```python
from build123d import *

# Parameters (mm, degrees)
BOSS_EXTRUDE33_DEPTH = 5
BOSS_EXTRUDE34_START = 5
BOSS_EXTRUDE34_DEPTH = 1
BOSS_EXTRUDE35_START = -4
BOSS_EXTRUDE35_DEPTH = 4
CUT_EXTRUDE2_DEPTH   = 35.891044696
CUT_EXTRUDE3_DEPTH   = 30.173146899
SKETCH22_W           = 13.5
SKETCH22_H           = 2
BOSS_EXTRUDE37_DEPTH = 1.75
SKETCH23_W           = 3
SKETCH23_H           = 3
BOSS_EXTRUDE38_DEPTH = 1.75
CUT_EXTRUDE4_DEPTH   = 3
CUT_EXTRUDE5_DEPTH   = 17.5


with BuildPart() as part:
    # lid → Boss-Extrude33 (new body)
    with BuildSketch(Plane(origin=(0, 0, 0), x_dir=(1, 0, 0), z_dir=(0, 1, 0))):
        with BuildLine():
            Line((-10.25, 23.85), (12.5, 23.85))
            ThreePointArc((12.5, 23.85), (13.207106781, 23.557106781), (13.5, 22.85))
            Line((13.5, 22.85), (13.5, -7.9))
            ThreePointArc((13.5, -7.9), (13.207106781, -8.607106781), (12.5, -8.9))
            Line((12.5, -8.9), (-10.25, -8.9))
            ThreePointArc((-10.25, -8.9), (-10.957106781, -8.607106781), (-11.25, -7.9))
            Line((-11.25, -7.9), (-11.25, 22.85))
            ThreePointArc((-11.25, 22.85), (-10.957106781, 23.557106781), (-10.25, 23.85))
        make_face()
        with BuildLine():
            Line((-10.5, 22.6), (-10.5, -7.65))
            ThreePointArc((-10.5, -7.65), (-10.353553391, -8.003553391), (-10, -8.15))
            Line((-10, -8.15), (12.25, -8.15))
            ThreePointArc((12.25, -8.15), (12.603553391, -8.003553391), (12.75, -7.65))
            Line((12.75, -7.65), (12.75, 22.6))
            ThreePointArc((12.75, 22.6), (12.603553391, 22.953553391), (12.25, 23.1))
            Line((12.25, 23.1), (-10, 23.1))
            ThreePointArc((-10, 23.1), (-10.353553391, 22.953553391), (-10.5, 22.6))
        make_face(mode=Mode.SUBTRACT)
    extrude(amount=BOSS_EXTRUDE33_DEPTH)

    # lid_5 → Boss-Extrude34 (add)
    with BuildSketch(Plane(origin=(0, 0, 0), x_dir=(1, 0, 0), z_dir=(0, 1, 0)).offset(BOSS_EXTRUDE34_START)):
        with BuildLine():
            Line((12.5, 23.85), (-10.25, 23.85))
            ThreePointArc((-10.25, 23.85), (-10.957106781, 23.557106781), (-11.25, 22.85))
            Line((-11.25, 22.85), (-11.25, -7.9))
            ThreePointArc((-11.25, -7.9), (-10.957106781, -8.607106781), (-10.25, -8.9))
            Line((-10.25, -8.9), (12.5, -8.9))
            ThreePointArc((12.5, -8.9), (13.207106781, -8.607106781), (13.5, -7.9))
            Line((13.5, -7.9), (13.5, 22.85))
            ThreePointArc((13.5, 22.85), (13.207106781, 23.557106781), (12.5, 23.85))
        make_face()
    extrude(amount=BOSS_EXTRUDE34_DEPTH)

    # lid_7 → Boss-Extrude35 (add)
    with BuildSketch(Plane(origin=(0, 0, 0), x_dir=(1, 0, 0), z_dir=(0, 1, 0)).offset(BOSS_EXTRUDE35_START)):
        with BuildLine():
            Line((-10.25, 23.85), (12.5, 23.85))
            ThreePointArc((12.5, 23.85), (13.207106781, 23.557106781), (13.5, 22.85))
            Line((13.5, 22.85), (13.5, -7.9))
            ThreePointArc((13.5, -7.9), (13.207106781, -8.607106781), (12.5, -8.9))
            Line((12.5, -8.9), (-10.25, -8.9))
            ThreePointArc((-10.25, -8.9), (-10.957106781, -8.607106781), (-11.25, -7.9))
            Line((-11.25, -7.9), (-11.25, 22.85))
            ThreePointArc((-11.25, 22.85), (-10.957106781, 23.557106781), (-10.25, 23.85))
        make_face()
        with BuildLine():
            Line((-10.5, 22.6), (-10.5, -7.65))
            ThreePointArc((-10.5, -7.65), (-10.353553391, -8.003553391), (-10, -8.15))
            Line((-10, -8.15), (12.25, -8.15))
            ThreePointArc((12.25, -8.15), (12.603553391, -8.003553391), (12.75, -7.65))
            Line((12.75, -7.65), (12.75, 22.6))
            ThreePointArc((12.75, 22.6), (12.603553391, 22.953553391), (12.25, 23.1))
            Line((12.25, 23.1), (-10, 23.1))
            ThreePointArc((-10, 23.1), (-10.353553391, 22.953553391), (-10.5, 22.6))
        make_face(mode=Mode.SUBTRACT)
    extrude(amount=BOSS_EXTRUDE35_DEPTH)

    # Sketch21 → Cut-Extrude2 (cut, through all)
    with BuildSketch(Plane(origin=(13.5, 0, 0), x_dir=(0, 0, -1), z_dir=(1, 0, 0))):
        with BuildLine():
            Line((4.05, 0), (4.05, -4))
            Line((4.05, -4), (10.05, -4))
            Line((10.05, -4), (10.05, 0))
            ThreePointArc((10.05, 0), (7.05, 3), (4.05, 0))
        make_face()
    extrude(amount=-CUT_EXTRUDE2_DEPTH, mode=Mode.SUBTRACT)

    # Sketch20 → Cut-Extrude3 (cut, through all)
    with BuildSketch(Plane(origin=(0, 6, 0), x_dir=(1, 0, 0), z_dir=(0, 1, 0))):
        with BuildLine():
            Line((-6.5, -3), (8.5, -3))
            ThreePointArc((8.5, -3), (10, -4.5), (8.5, -6))
            Line((8.5, -6), (-6.5, -6))
            ThreePointArc((-6.5, -6), (-8, -4.5), (-6.5, -3))
        make_face()
    extrude(amount=-CUT_EXTRUDE3_DEPTH, mode=Mode.SUBTRACT)

    # Sketch22 → Boss-Extrude37 (add)
    with BuildSketch(Plane(origin=(0, 0, 8.15), x_dir=(-1, 0, 0), z_dir=(0, 0, -1))):
        with Locations((-0.75, -3)):
            Rectangle(SKETCH22_W, SKETCH22_H)
    extrude(amount=BOSS_EXTRUDE37_DEPTH)

    # Sketch23 → Boss-Extrude38 (add)
    with BuildSketch(Plane.XY.offset(-23.1)):
        with Locations((-7.5, -2.5)):
            Rectangle(SKETCH23_W, SKETCH23_H)
        with Locations((9.75, -2.5)):
            Rectangle(SKETCH23_W, SKETCH23_H)
    extrude(amount=BOSS_EXTRUDE38_DEPTH)

    # Sketch24 → Cut-Extrude4 (cut)
    with BuildSketch(Plane.ZY.offset(-8.25)):
        Polygon((-23.1, -4), (-21.35, -1), (-21.35, -4), align=None)
    extrude(amount=-CUT_EXTRUDE4_DEPTH, mode=Mode.SUBTRACT)

    # Sketch24_2 → Cut-Extrude5 (cut)
    with BuildSketch(Plane.ZY.offset(-8.25)):
        Polygon((-23.1, -4), (-21.35, -1), (-21.35, -4), align=None)
    extrude(amount=CUT_EXTRUDE5_DEPTH, mode=Mode.SUBTRACT)


solid = part.part
```
Model file for the job. Use its own axes, mm. A direction names the side the tool comes from. Coordinates: 2 decimals unless noted, no trailing zeros. Write each loop counter-clockwise with the first axis right and the second up, starting at its lowest first coordinate (ties: lowest second). Pieces come first, ordered by that corner, then holes. Notation, with made-up numbers: (3.5, 9.25) - (18.5, 9.25) arc R16 ccw to (18.5, 24.25) - close; hole circle Ø7 at (34, 75). An arc over 180 degrees is marked (long way). One line per item, written item: value. Start each with the question number.
1. Slice it at D-D (z = -7.05). Write the cut outline in (x, y), plus the area to 4 significant figures.
2. Mould opens along Z. For faces 1 (the cylindrical face through (-10.965, 0.93, -23.549)), 2 (the cylindrical face through (-10.949, 0.93, 8.615)), 3 (the flat face through (-9, -1.9, -22.6)), 4 (the flat face through (13.5, 3.2, -7.7)) say: released by +Z, released by -Z, zero draft, split by the parting line, or undercut.
3. Probe line 1 (X direction, y = 3.25, z = -8); line 2 (Z direction, x = 2, y = -1.5); line 3 (Z direction, x = 4.75, y = -2.75). List the from-to ranges inside material, lowest first. Write a range as from..to.
4. Slice it at C-C (z = 4.5). Write the cut outline in (x, y), plus the area to 4 significant figures.
5. Tool access for faces 5 (the flat face through (1, 1, -23.1)), 6 (the flat face through (1, 1, -23.85)), 7 (the flat face through (1.2, -4, -23.6)), 8 (the flat face through (0.9, 5.5, 3)), 9 (the flat face through (-10.5, 3.4, -7.7)): list every direction of +Z, -Z, +X, -X, +Y, -Y with a clear straight run to the whole face (end or side of a thin tool).
6. Slice it at A-A (x = -0.25). Write the cut outline in (y, z).
7. Slice it at B-B (y = 4). Write the cut outline in (x, z).
8. Flat gauge pin, fed straight in: pin 1 (1.5 mm diameter, centred on x = 3.5, z = -4.5, fed in from -Y). Where does the tip first touch, or does it go through?
Answers below:
1. outline: (-11.25, 3) - (-10.5, 3) - (-10.5, 5) - (12.75, 5) - (12.75, 3) - (13.5, 3) - (13.5, 6) - (-11.25, 6) - close
1. area: 27.75 mm^2
2. face 1: released by -Z
2. face 2: released by +Z
2. face 3: undercut
2. face 4: zero draft
3. line 1: x = -11.25..-10.5, 12.75..13.5
3. line 2: z = -23.85..-23.1, 8.15..8.9
3. line 3: z = -23.85..-23.1, 6.4..8.9
4. outline: (-11.25, -4) - (-10.5, -4) - (-10.5, 5) - (-8, 5) - (-8, 6) - (-11.25, 6) - close; (10, 5) - (12.75, 5) - (12.75, -4) - (13.5, -4) - (13.5, 6) - (10, 6) - close
4. area: 20.25 mm^2
5. face 5: none
5. face 6: -Z, +X, -X, +Y, -Y
5. face 7: +Z, -Z, +X, -X, -Y
5. face 8: +Y, -Y
5. face 9: -Y
6. outline: (-4, -23.85) - (6, -23.85) - (6, 3) - (5, 3) - (5, -23.1) - (-4, -23.1) - close; (-4, 6.4) - (-2, 6.4) - (-2, 8.15) - (5, 8.15) - (5, 6) - (6, 6) - (6, 8.9) - (-4, 8.9) - close
7. outline: (-11.25, -22.85) arc R1 ccw to (-10.25, -23.85) - (12.5, -23.85) arc R1 ccw to (13.5, -22.85) - (13.5, 7.9) arc R1 ccw to (12.5, 8.9) - (-10.25, 8.9) arc R1 ccw to (-11.25, 7.9) - close; hole (-10.5, -22.6) arc R0.5 ccw to (-10, -23.1) - (12.25, -23.1) arc R0.5 ccw to (12.75, -22.6) - (12.75, 7.65) arc R0.5 ccw to (12.25, 8.15) - (-10, 8.15) arc R0.5 ccw to (-10.5, 7.65) - close
8. pin 1: stops at y = 5
